Design review of the part built by this model. Coordinates are the model's own, in mm. A direction names the side the tool comes from. Give positions to 0.01 mm unless a question says otherwise; leave off trailing zeros. Order: outer loops, then holes, each group sorted by start corner. A loop starts at its lowest first (then second) coordinate and runs counter-clockwise, first axis right, second up. Notation, with made-up numbers: (13.25, 84.5) -> (19.25, 84.5) arc R27 ccw to (19.25, 119.5) -> close; hole circle Ø7 at (45.5, -0.75). An arc over 180 degrees is marked (long way). One line per item, written item: value. Start each with the question number.
1) Wall thickness on line 1 along Y through (x, z) = (75, 7.5); line 2 along Z through (x, y) = (17, 18); line 3 along X through (y, z) = (2, 9.75): over which ranges is each line inside the solid? List them lowest first. Write a range as from..to.
2) For pin 1 (1.5 mm diameter, centred on y = 4, z = 8.5, fed in from +X); pin 2 (1.5 mm diameter, centred on x = 57, z = 4, fed in from +Y); pin 3 (2 mm diameter, centred on y = 32, z = 9, fed in from -X), all flat-tipped, find the tip position at first contact; note any pin that passes through.
3) Consider section A-A (z = 10.25). State the section outline as (x, y) points, plus the area to 3 significant figures.
4) Consider section C-C (x = -29.5). State the section outline as (y, z) points, plus the area to 3 significant figures.
5) Consider section B-B (z = 1.75). State how many separate pieces and enclosed holes the cut face has, plus the area to 3 significant figures.
6) Tool access review of faces 4 (the face through (-28, 4, 12.4)), 5 (the face through (-50.4, 14.7, 2.5)), 6 (the face through (-73.32, 28.76, 8.85)): name each direction out of +Z, -Z, +X, -X, +Y, -Y from which nothing blocks a thin tool from reaching the whole face with its end or side.
7) Consider section D-D (x = 42). State the section outline as (y, z) points, plus the area to 3 significant figures.
8) The part is to be moulded in two halves that separate along X. For faces 1 (the face through (0, 19, 0)), 2 (the face through (23.685, -3.243, 6.113)), 3 (the face through (-29.6, 4, 6.1)), say which applies: released by +X, released by -X, zero draft, split by the parting line, or undercut.
from build123d import *

# Parameters (mm, degrees)
F0_R     = 1.6
F1_DEPTH = 5
F2_R     = 5.65
F2_R_2   = 1.6
F3_DEPTH = 0.4
F4_R     = 3.65
F4_R_2   = 1.6
F5_DEPTH = 7
F7_DEPTH = 7.4


with BuildPart() as f1:
    # F0 (on Top) → F1 (new body)
    with BuildSketch(Plane.XY):
        with BuildLine():
            ThreePointArc((-37.3521878639, -1.5307337295), (-35.273852997, -3.2430337771), (-33.19551813, -1.5307337295))
            ThreePointArc((-33.19551813, -1.5307337295), (-29.5, 4), (-25.80448187, -1.5307337295))
            ThreePointArc((-25.80448187, -1.5307337295), (-23.726147003, -3.2430337771), (-21.6478121361, -1.5307337295))
            ThreePointArc((-21.6478121361, -1.5307337295), (-21.537038776, -0.7689268785), (-21.5, 0))
            ThreePointArc((-21.5, 0), (0, 15), (21.5, 0))
            ThreePointArc((21.5, 0), (21.537038776, -0.7689268785), (21.6478121361, -1.5307337295))
            ThreePointArc((21.6478121361, -1.5307337295), (23.726147003, -3.2430337771), (25.80448187, -1.5307337295))
            ThreePointArc((25.80448187, -1.5307337295), (29.5, 4), (33.19551813, -1.5307337295))
            ThreePointArc((33.19551813, -1.5307337295), (35.273852997, -3.2430337771), (37.3521878639, -1.5307337295))
            ThreePointArc((37.3521878639, -1.5307337295), (37.4352026436, -1.0161491059), (37.4845313984, -0.4972507899))
            Line((37.4845313984, -0.4972507899), (68.9534299936, 21.6347218485))
            ThreePointArc((68.9534299936, 21.6347218485), (71.8681744795, 20.4158872196), (75, 20))
            ThreePointArc((75, 20), (83.4852813742, 40.4852813742), (63, 32))
            ThreePointArc((63, 32), (0, 20), (-63, 32))
            ThreePointArc((-63, 32), (-83.4852813742, 40.4852813742), (-75, 20))
            ThreePointArc((-75, 20), (-71.8681744795, 20.4158872196), (-68.9534299936, 21.6347218485))
            Line((-68.9534299936, 21.6347218485), (-37.4845313984, -0.4972507899))
            ThreePointArc((-37.4845313984, -0.4972507899), (-37.4352026436, -1.0161491059), (-37.3521878639, -1.5307337295))
        make_face()
        with BuildLine():
            ThreePointArc((-65.1844431468, 25.0967512241), (-64.5810704237, 26.0463535136), (-64.0692832138, 27.0482901398))
            ThreePointArc((-64.0692832138, 27.0482901398), (-43.3702293382, 20.4154614181), (-22.0125035411, 16.3790277239))
            ThreePointArc((-22.0125035411, 16.3790277239), (-19.5611083836, 14.4098541759), (-20.2140176404, 11.3340303541))
            ThreePointArc((-20.2140176404, 11.3340303541), (-22.3670470232, 8.782690509), (-24.2000278476, 5.9925199361))
            ThreePointArc((-24.2000278476, 5.9925199361), (-30.4327318488, 7.9454396542), (-36.0437045688, 4.6021658506))
            Line((-36.0437045688, 4.6021658506), (-65.1844431468, 25.0967512241))
        make_face(mode=Mode.SUBTRACT)
        with BuildLine():
            ThreePointArc((20.2140176404, 11.3340303541), (19.5611083836, 14.4098541759), (22.0125035411, 16.3790277239))
            ThreePointArc((22.0125035411, 16.3790277239), (43.3702293382, 20.4154614181), (64.0692832138, 27.0482901398))
            ThreePointArc((64.0692832138, 27.0482901398), (64.5810704237, 26.0463535136), (65.1844431468, 25.0967512241))
            Line((65.1844431468, 25.0967512241), (36.0437045688, 4.6021658506))
            ThreePointArc((36.0437045688, 4.6021658506), (30.4327318488, 7.9454396542), (24.2000278476, 5.9925199361))
            ThreePointArc((24.2000278476, 5.9925199361), (22.3670470232, 8.782690509), (20.2140176404, 11.3340303541))
        make_face(mode=Mode.SUBTRACT)
        with Locations((-75, 32)):
            Circle(F0_R, mode=Mode.SUBTRACT)
        with Locations((75, 32)):
            Circle(F0_R, mode=Mode.SUBTRACT)
    extrude(amount=F1_DEPTH)

    # F2 (on face) → F3 (join)
    with BuildSketch(Plane.XY.offset(5)):
        with Locations((-75, 32)):
            Circle(F2_R)
        with Locations((-75, 32)):
            Circle(F2_R_2, mode=Mode.SUBTRACT)
        with Locations((75, 32)):
            Circle(F2_R)
        with Locations((75, 32)):
            Circle(F2_R_2, mode=Mode.SUBTRACT)
    extrude(amount=F3_DEPTH)

    # F4 (on face) → F5 (join)
    with BuildSketch(Plane.XY.offset(5.4)):
        with Locations((-75, 32)):
            Circle(F4_R)
        with Locations((-75, 32)):
            Circle(F4_R_2, mode=Mode.SUBTRACT)
        with Locations((75, 32)):
            Circle(F4_R)
        with Locations((75, 32)):
            Circle(F4_R_2, mode=Mode.SUBTRACT)
    extrude(amount=F5_DEPTH)

    # F6 (on face) → F7 (join, through all)
    with BuildSketch(Plane.XY.offset(5)):
        with BuildLine():
            ThreePointArc((-21.6478121361, -1.5307337295), (-29.5, 8), (-37.3521878639, -1.5307337295))
            ThreePointArc((-37.3521878639, -1.5307337295), (-35.273852997, -3.2430337771), (-33.19551813, -1.5307337295))
            ThreePointArc((-33.19551813, -1.5307337295), (-29.5, 4), (-25.80448187, -1.5307337295))
            ThreePointArc((-25.80448187, -1.5307337295), (-23.726147003, -3.2430337771), (-21.6478121361, -1.5307337295))
        make_face()
        with BuildLine():
            ThreePointArc((37.3521878639, -1.5307337295), (29.5, 8), (21.6478121361, -1.5307337295))
            ThreePointArc((21.6478121361, -1.5307337295), (23.726147003, -3.2430337771), (25.80448187, -1.5307337295))
            ThreePointArc((25.80448187, -1.5307337295), (29.5, 4), (33.19551813, -1.5307337295))
            ThreePointArc((33.19551813, -1.5307337295), (35.273852997, -3.2430337771), (37.3521878639, -1.5307337295))
        make_face()
    extrude(amount=F7_DEPTH)


solid = f1.part
Checked values:
1. line 1: y = 28.35..30.4, 33.6..35.65
1. line 2: z = 0..5
1. line 3: x = -37.25..-32.96, -26.04..-21.75, 21.75..26.04, 32.96..37.25
2. pin 1: stops at x = 36.81
2. pin 2: stops at y = 30.02
2. pin 3: stops at x = -78.65
3. outline: circle Ø7.3 at (-75, 32); (-37.35, -1.53) arc R2.12 ccw to (-33.2, -1.53) arc R4 cw (long way) to (-25.8, -1.53) arc R2.12 ccw to (-21.65, -1.53) arc R8 ccw (long way) to start; (21.65, -1.53) arc R2.12 ccw to (25.8, -1.53) arc R4 cw (long way) to (33.2, -1.53) arc R2.12 ccw to (37.35, -1.53) arc R8 ccw (long way) to start; circle Ø7.3 at (75, 32); hole circle Ø3.2 at (-75, 32); hole circle Ø3.2 at (75, 32)
3. area: 265 mm^2
4. outline: (4, 0) -> (8, 0) -> (8, 12.4) -> (4, 12.4) -> close; (17.48, 0) -> (22.56, 0) -> (22.56, 5) -> (17.48, 5) -> close
4. area: 75.0 mm^2
5. separate pieces: 1
5. enclosed holes: 4
5. area: 2,300 mm^2
6. face 4: +Z, +X, -X, +Y, -Y
6. face 5: +Z, -Z
6. face 6: +Z
7. outline: (2.68, 0) -> (8.79, 0) -> (8.79, 5) -> (2.68, 5) -> close; (20.07, 0) -> (25.23, 0) -> (25.23, 5) -> (20.07, 5) -> close
7. area: 56.3 mm^2
8. face 1: zero draft
8. face 2: undercut
8. face 3: undercut
